Check sheet for the modelled part. Datum: model origin and axes. Units: mm. A direction names the side the tool comes from. Give positions to 0.01 mm unless a question says otherwise; leave off trailing zeros. Loops run counter-clockwise (first coordinate to the right, second up) from the corner with the lowest first, then second, coordinate; pieces in that order, holes last. Notation, with made-up numbers: (-1.75, 4.5) - (46.25, 4.5) arc R26 ccw to (46.25, 39.5) - close; hole circle Ø5 at (70, -29.5). An arc over 180 degrees is marked (long way). Answer in a Markdown table with one row per item. Add a question column.
(1) Draft check along X on faces 1 (the face through (2, 9.9, -19.5)), 2 (the face through (2.788, -3.834, -13.421)), 3 (the face through (20.963, -24.725, 26.859)), 4 (the face through (54.324, -24.725, -82.987)). Enter one of: released by +X, released by -X, zero draft, split by the parting line, or undercut.
(2) Set-up check for faces 5 (the face through (56, -23.76, 4)), 6 (the face through (3, 2.74, -55)), 7 (the face through (46, -22.26, -14)): record each of +Z, -Z, +X, -X, +Y, -Y from which the full face is reachable in a straight line by a thin tool's end or side.
(3) Sectioned sample at D-D on y = -3.26. Enter the section's corners in (x, z) (3 decimals), then the cut area to 3 significant figures.
(4) Go/stop test with flat-tipped pins: P1, Ø6, axis at y = 14, z = 6.5, coming from the +X side; P2, Ø6, axis at y = 11.26, z = 20.925, coming from the -X side; P3, Ø2, axis at x = 73, y = -24.5, coming from the +Z side; P4, Ø6, axis at x = 7.5, y = 52, coming from the -Z side (3 decimals). Record where each tip stops, or that it passes through.
(5) Thickness scan on L1, parallel to Z at x = 1, y = 54 (3 decimals); L2, parallel to Z at x = 62.5, y = -22.5 (3 decimals); L3, parallel to X at y = 9, z = -89. Record the ranges inside material, lowest first.
(6) Sectioned sample at A-A on x = 35.5. Enter the section's corners in (y, z) (3 decimals).
(7) Sectioned sample at C-C on z = -60. Enter the section's corners in (x, y) (3 decimals), then the cut area to 3 significant figures.
(8) Sectioned sample at B-B on y = 11.26. Enter the section's corners in (x, z) (3 decimals), then the cut area to 3 significant figures.
from build123d import *

# Parameters (mm, degrees)
SKETCH_1_W          = 125
SKETCH_1_H          = 92.025
SKETCH_1_R          = 1.75
SKETCH_1_R_2        = 1.5
SKETCH_1_W_2        = 29.91
SKETCH_1_H_2        = 21.53
SKETCH_1_W_3        = 29.85
SKETCH_1_H_3        = 10.52
SKETCH_1_W_4        = 34.33
SKETCH_1_H_4        = 41.73
EXTRUDE_1_DEPTH     = 5.5
FILLET_1_R          = 5
SKETCH_2_R          = 3
SKETCH_2_R_2        = 1.5
SKETCH_2_R_3        = 3.25
SKETCH_2_R_4        = 1.75
CUT_EXTRUDE_1_DEPTH = 2
SKETCH_3_W          = 86.5
SKETCH_3_H          = 125
SKETCH_3_W_2        = 38
SKETCH_3_H_2        = 50
SKETCH_3_R          = 1.5
EXTRUDE_2_DEPTH     = 5
SKETCH_6_R          = 3
SKETCH_6_R_2        = 1.5
CUT_EXTRUDE_2_DEPTH = 1.5
FILLET_3_R          = 7
FILLET_4_R          = 10
SKETCH_7_W          = 5.5
SKETCH_7_H          = 92.025
EXTRUDE_5_DEPTH     = 20
FILLET_6_R          = 5
EXTRUDE_6_DEPTH     = 20
FILLET_5_R          = 10


with BuildPart() as part:
    # 草图1 → 凸台-拉伸1 (new body)
    with BuildSketch(Plane(origin=(0, 0, 0), x_dir=(0, 0, -1), z_dir=(1, 0, 0))):
        with Locations((28.575, 23.7525)):
            Rectangle(SKETCH_1_W, SKETCH_1_H)
        with Locations((-20.925, 11.26)):
            Circle(SKETCH_1_R, mode=Mode.SUBTRACT)
        with Locations((20.925, 11.26)):
            Circle(SKETCH_1_R, mode=Mode.SUBTRACT)
        with Locations((20.925, -11.26)):
            Circle(SKETCH_1_R, mode=Mode.SUBTRACT)
        with Locations((-20.925, -11.26)):
            Circle(SKETCH_1_R, mode=Mode.SUBTRACT)
        with Locations((-20.955, 56.765)):
            Circle(SKETCH_1_R, mode=Mode.SUBTRACT)
        with Locations((20.955, 56.765)):
            Circle(SKETCH_1_R, mode=Mode.SUBTRACT)
        with Locations((20.955, 23.235)):
            Circle(SKETCH_1_R, mode=Mode.SUBTRACT)
        with Locations((-20.955, 23.235)):
            Circle(SKETCH_1_R, mode=Mode.SUBTRACT)
        with Locations((31.835, 50.47)):
            Circle(SKETCH_1_R, mode=Mode.SUBTRACT)
        with Locations((78.165, 50.47)):
            Circle(SKETCH_1_R, mode=Mode.SUBTRACT)
        with Locations((78.165, -3.26)):
            Circle(SKETCH_1_R, mode=Mode.SUBTRACT)
        with Locations((31.835, -3.26)):
            Circle(SKETCH_1_R, mode=Mode.SUBTRACT)
        with Locations((-28.925, 64.765)):
            Circle(SKETCH_1_R_2, mode=Mode.SUBTRACT)
        with Locations((86.075, 64.765)):
            Circle(SKETCH_1_R_2, mode=Mode.SUBTRACT)
        with Locations((0, 40)):
            Rectangle(SKETCH_1_W_2, SKETCH_1_H_2, mode=Mode.SUBTRACT)
        Rectangle(SKETCH_1_W_3, SKETCH_1_H_3, mode=Mode.SUBTRACT)
        with Locations((55, 23.605)):
            Rectangle(SKETCH_1_W_4, SKETCH_1_H_4, mode=Mode.SUBTRACT)
    extrude(amount=EXTRUDE_1_DEPTH)

    # 圆角1
    fillet_1_edges = [part.edges().sort_by_distance(p)[0] for p in [
        (2.75, 50.765, 14.955),
        (2.75, 29.235, 14.955),
        (2.75, 29.235, -14.955),
        (2.75, 50.765, -14.955),
        (2.75, 5.26, -14.925),
        (2.75, 5.26, 14.925),
        (2.75, -5.26, 14.925),
        (2.75, -5.26, -14.925),
        (2.75, 44.47, -72.165),
        (2.75, 44.47, -37.835),
        (2.75, 2.74, -37.835),
        (2.75, 2.74, -72.165),
    ]]
    fillet(fillet_1_edges, radius=FILLET_1_R)

    # 草图2 → 切除-拉伸1 (cut)
    # profile 1 of 14: a face of its own
    with BuildSketch(Plane.ZY):
        with Locations((-86.075, 64.765)):
            Circle(SKETCH_2_R)
        with Locations((-86.075, 64.765)):
            Circle(SKETCH_2_R_2, mode=Mode.SUBTRACT)
    # profile 2 of 14: a face of its own
    with BuildSketch(Plane.ZY):
        with Locations((-78.165, 50.47)):
            Circle(SKETCH_2_R_3)
        with Locations((-78.165, 50.47)):
            Circle(SKETCH_2_R_4, mode=Mode.SUBTRACT)
    # profile 3 of 14: a face of its own
    with BuildSketch(Plane.ZY):
        with Locations((-31.835, 50.47)):
            Circle(SKETCH_2_R_3)
        with Locations((-31.835, 50.47)):
            Circle(SKETCH_2_R_4, mode=Mode.SUBTRACT)
    # profile 4 of 14: a face of its own
    with BuildSketch(Plane.ZY):
        with Locations((-78.165, -3.26)):
            Circle(SKETCH_2_R_3)
        with Locations((-78.165, -3.26)):
            Circle(SKETCH_2_R_4, mode=Mode.SUBTRACT)
    # profile 5 of 14: a face of its own
    with BuildSketch(Plane.ZY):
        with Locations((-31.835, -3.26)):
            Circle(SKETCH_2_R_3)
        with Locations((-31.835, -3.26)):
            Circle(SKETCH_2_R_4, mode=Mode.SUBTRACT)
    # profile 6 of 14: a face of its own
    with BuildSketch(Plane.ZY):
        with Locations((-20.925, -11.26)):
            Circle(SKETCH_2_R_3)
        with Locations((-20.925, -11.26)):
            Circle(SKETCH_2_R_4, mode=Mode.SUBTRACT)
    # profile 7 of 14: a face of its own
    with BuildSketch(Plane.ZY):
        with Locations((-20.955, 23.235)):
            Circle(SKETCH_2_R_3)
        with Locations((-20.955, 23.235)):
            Circle(SKETCH_2_R_4, mode=Mode.SUBTRACT)
    # profile 8 of 14: a face of its own
    with BuildSketch(Plane.ZY):
        with Locations((-20.925, 11.26)):
            Circle(SKETCH_2_R_3)
        with Locations((-20.925, 11.26)):
            Circle(SKETCH_2_R_4, mode=Mode.SUBTRACT)
    # profile 9 of 14: a face of its own
    with BuildSketch(Plane.ZY):
        with Locations((20.955, 56.765)):
            Circle(SKETCH_2_R_3)
        with Locations((20.955, 56.765)):
            Circle(SKETCH_2_R_4, mode=Mode.SUBTRACT)
    # profile 10 of 14: a face of its own
    with BuildSketch(Plane.ZY):
        with Locations((28.925, 64.765)):
            Circle(SKETCH_2_R)
        with Locations((28.925, 64.765)):
            Circle(SKETCH_2_R_2, mode=Mode.SUBTRACT)
    # profile 11 of 14: a face of its own
    with BuildSketch(Plane.ZY):
        with Locations((20.955, 23.235)):
            Circle(SKETCH_2_R_3)
        with Locations((20.955, 23.235)):
            Circle(SKETCH_2_R_4, mode=Mode.SUBTRACT)
    # profile 12 of 14: a face of its own
    with BuildSketch(Plane.ZY):
        with Locations((20.925, 11.26)):
            Circle(SKETCH_2_R_3)
        with Locations((20.925, 11.26)):
            Circle(SKETCH_2_R_4, mode=Mode.SUBTRACT)
    # profile 13 of 14: a face of its own
    with BuildSketch(Plane.ZY):
        with Locations((20.925, -11.26)):
            Circle(SKETCH_2_R_3)
        with Locations((20.925, -11.26)):
            Circle(SKETCH_2_R_4, mode=Mode.SUBTRACT)
    # profile 14 of 14: a face of its own
    with BuildSketch(Plane.ZY):
        with Locations((-20.955, 56.765)):
            Circle(SKETCH_2_R_3)
    extrude(amount=-CUT_EXTRUDE_1_DEPTH, mode=Mode.SUBTRACT)

    # 草图3 → 凸台-拉伸2 (add)
    with BuildSketch(Plane.XZ.offset(22.26)):
        with Locations((37.25, -28.575)):
            Rectangle(SKETCH_3_W, SKETCH_3_H)
        with BuildLine():
            ThreePointArc((50.325, -79.075), (54.325, -83.075), (50.325, -87.075))
            Line((50.325, -87.075), (20.325, -87.075))
            ThreePointArc((20.325, -87.075), (16.325, -83.075), (20.325, -79.075))
            Line((20.325, -79.075), (50.325, -79.075))
        make_face(mode=Mode.SUBTRACT)
        with Locations((35.325, -42.922390802)):
            Rectangle(SKETCH_3_W_2, SKETCH_3_H_2, mode=Mode.SUBTRACT)
        with Locations(Location((65.94, -71.075, 0), (0, 0, 270))):
            Circle(SKETCH_3_R, mode=Mode.SUBTRACT)
        with BuildLine():
            ThreePointArc((71.5, -10.075), (69.5, -8.075), (71.5, -6.075))
            Line((71.5, -6.075), (75.5, -6.075))
            ThreePointArc((75.5, -6.075), (77.5, -8.075), (75.5, -10.075))
            Line((75.5, -10.075), (75.5, -47.075))
            ThreePointArc((75.5, -47.075), (77.5, -49.075), (75.5, -51.075))
            Line((75.5, -51.075), (71.5, -51.075))
            ThreePointArc((71.5, -51.075), (69.5, -49.075), (71.5, -47.075))
            Line((71.5, -47.075), (71.5, -10.075))
        make_face(mode=Mode.SUBTRACT)
        with Locations(Location((16.5, 3.335, 0), (0, 0, 270))):
            Circle(SKETCH_3_R, mode=Mode.SUBTRACT)
        with Locations(Location((54.15, 3.335, 0), (0, 0, 270))):
            Circle(SKETCH_3_R, mode=Mode.SUBTRACT)
        with BuildLine():
            ThreePointArc((63.961913607, 29.925), (66.961913607, 26.925), (63.961913607, 23.925))
            Line((63.961913607, 23.925), (23.961913607, 23.925))
            ThreePointArc((23.961913607, 23.925), (20.961913607, 26.925), (23.961913607, 29.925))
            Line((23.961913607, 29.925), (63.961913607, 29.925))
        make_face(mode=Mode.SUBTRACT)
    extrude(amount=EXTRUDE_2_DEPTH)

    # 草图6 → 切除-拉伸2 (cut)
    # profile 1 of 3: a face of its own
    with BuildSketch(Plane(origin=(0, -22.26, 0), x_dir=(1, 0, 0), z_dir=(0, 1, 0))):
        with Locations(Location((65.94, 71.075, 0), (0, 0, 270))):
            Circle(SKETCH_6_R)
        with Locations(Location((65.94, 71.075, 0), (0, 0, 270))):
            Circle(SKETCH_6_R_2, mode=Mode.SUBTRACT)
    # profile 2 of 3: a face of its own
    with BuildSketch(Plane(origin=(0, -22.26, 0), x_dir=(1, 0, 0), z_dir=(0, 1, 0))):
        with Locations(Location((54.15, -3.335, 0), (0, 0, 270))):
            Circle(SKETCH_6_R)
        with Locations(Location((54.15, -3.335, 0), (0, 0, 270))):
            Circle(SKETCH_6_R_2, mode=Mode.SUBTRACT)
    # profile 3 of 3: a face of its own
    with BuildSketch(Plane(origin=(0, -22.26, 0), x_dir=(1, 0, 0), z_dir=(0, 1, 0))):
        with Locations(Location((16.5, -3.335, 0), (0, 0, 270))):
            Circle(SKETCH_6_R)
        with Locations(Location((16.5, -3.335, 0), (0, 0, 270))):
            Circle(SKETCH_6_R_2, mode=Mode.SUBTRACT)
    extrude(amount=-CUT_EXTRUDE_2_DEPTH, mode=Mode.SUBTRACT)

    # 圆角3
    fillet_3_edges = [part.edges().sort_by_distance(p)[0] for p in [
        (5.5, -22.26, -28.575),
    ]]
    fillet(fillet_3_edges, radius=FILLET_3_R)

    # 圆角4
    fillet_4_edges = [part.edges().sort_by_distance(p)[0] for p in [
        (80.5, -24.76, -91.075),
        (80.5, -24.76, 33.925),
    ]]
    fillet(fillet_4_edges, radius=FILLET_4_R)

    # 草图7 → 凸台-拉伸5 (add)
    with BuildSketch(Plane.XY.offset(33.925)):
        with Locations((2.75, 23.7525)):
            Rectangle(SKETCH_7_W, SKETCH_7_H)
    extrude(amount=EXTRUDE_5_DEPTH)

    # 圆角6
    fillet_6_edges = [part.edges().sort_by_distance(p)[0] for p in [
        (-6, -24.76, -91.075),
        (16.325, -24.76, -67.922390802),
        (16.325, -24.76, -17.922390802),
        (54.325, -24.76, -17.922390802),
        (-6, -24.76, 33.925),
        (54.325, -24.76, -67.922390802),
    ]]
    fillet(fillet_6_edges, radius=FILLET_6_R)

    # 草图8 → 凸台-拉伸6 (add)
    with BuildSketch(Plane(origin=(0, 0, -91.075), x_dir=(-1, 0, 0), z_dir=(0, 0, -1))):
        Polygon((-5.5, -22.26), (-5.5, -15.26), (-5.5, 69.765), (0, 69.765), (0, -22.26), align=None)
    extrude(amount=EXTRUDE_6_DEPTH)

    # 圆角5
    fillet_5_edges = [part.edges().sort_by_distance(p)[0] for p in [
        (2.75, -22.26, 53.925),
        (2.75, 69.765, 53.925),
        (2.75, -22.26, -111.075),
        (2.75, 69.765, -111.075),
    ]]
    fillet(fillet_5_edges, radius=FILLET_5_R)


solid = part.part
Reply:
| question | item | result |
|---|---|---|
| 1 | face 1 | released by -X |
| 1 | face 2 | zero draft |
| 1 | face 3 | undercut |
| 1 | face 4 | undercut |
| 2 | face 5 | +Y |
| 2 | face 6 | +X, -X |
| 2 | face 7 | +Z, -Z, +X, +Y |
| 3 | outline | (0, -111.075) - (5.5, -111.075) - (5.5, -79.915) - (2, -79.915) - (2, -81.415) - (0, -81.415) - close; (0, -74.915) - (2, -74.915) - (2, -76.415) - (5.5, -76.415) - (5.5, -33.585) - (2, -33.585) - (2, -35.085) - (0, -35.085) - close; (0, -28.585) - (2, -28.585) - (2, -30.085) - (5.5, -30.085) - (5.5, -13.925) - (0, -13.925) - close; (0, 13.925) - (5.5, 13.925) - (5.5, 53.925) - (0, 53.925) - close |
| 3 | area | 704 mm^2 |
| 4 | P1 | x = 5.5 |
| 4 | P2 | x = 2 |
| 4 | P3 | z = 33.81 |
| 4 | P4 | z = -111.075 |
| 5 | L1 | -111.075 to -22.663, -19.247 to 19.247, 22.663 to 53.925 |
| 5 | L2 | -91.075 to 23.925, 29.925 to 33.925 |
| 5 | L3 | 0 to 5.5 |
| 6 | outline | (-27.26, -91.075) - (-22.26, -91.075) - (-22.26, -87.075) - (-27.26, -87.075) - close; (-27.26, -79.075) - (-22.26, -79.075) - (-22.26, -67.922) - (-27.26, -67.922) - close; (-27.26, -17.922) - (-22.26, -17.922) - (-22.26, 23.925) - (-27.26, 23.925) - close; (-27.26, 29.925) - (-22.26, 29.925) - (-22.26, 33.925) - (-27.26, 33.925) - close |
| 7 | outline | (-6, -27.26) - (16.325, -27.26) - (16.325, -22.26) - (12.5, -22.26) arc R7 cw to (5.5, -15.26) - (5.5, 2.74) - (0, 2.74) - (0, -22.26) - (-6, -22.26) - close; (0, 44.47) - (5.5, 44.47) - (5.5, 69.765) - (0, 69.765) - close; (54.325, -27.26) - (80.5, -27.26) - (80.5, -22.26) - (54.325, -22.26) - close |
| 7 | area | 530 mm^2 |
| 8 | outline | (0, -111.075) - (5.5, -111.075) - (5.5, -72.165) - (0, -72.165) - close; (0, -37.835) - (5.5, -37.835) - (5.5, -22.675) - (2, -22.675) - (2, -24.175) - (0, -24.175) - close; (0, -17.675) - (2, -17.675) - (2, -19.175) - (5.5, -19.175) - (5.5, 19.175) - (2, 19.175) - (2, 17.675) - (0, 17.675) - close; (0, 24.175) - (2, 24.175) - (2, 22.675) - (5.5, 22.675) - (5.5, 53.925) - (0, 53.925) - close |
| 8 | area | 668 mm^2 |
